Design review of the part shown in the three views and the two pictorial views. Dimensions are in mm from the part's minimum x, y and z. A direction names the side the tool comes from. Round coordinates to 2 decimals unless told otherwise and drop trailing zeros. Loops run counter-clockwise (first coordinate to the right, second up) from the corner with the lowest first, then second, coordinate; pieces in that order, holes last. Notation, with made-up numbers: M 75,-33.75 L 117,-33.75 A6 ccw 117,-24.75 Z; hole C -11,35 d2. An arc over 180 degrees is marked long. Answer in a Markdown table with one row per item. Add a question column.
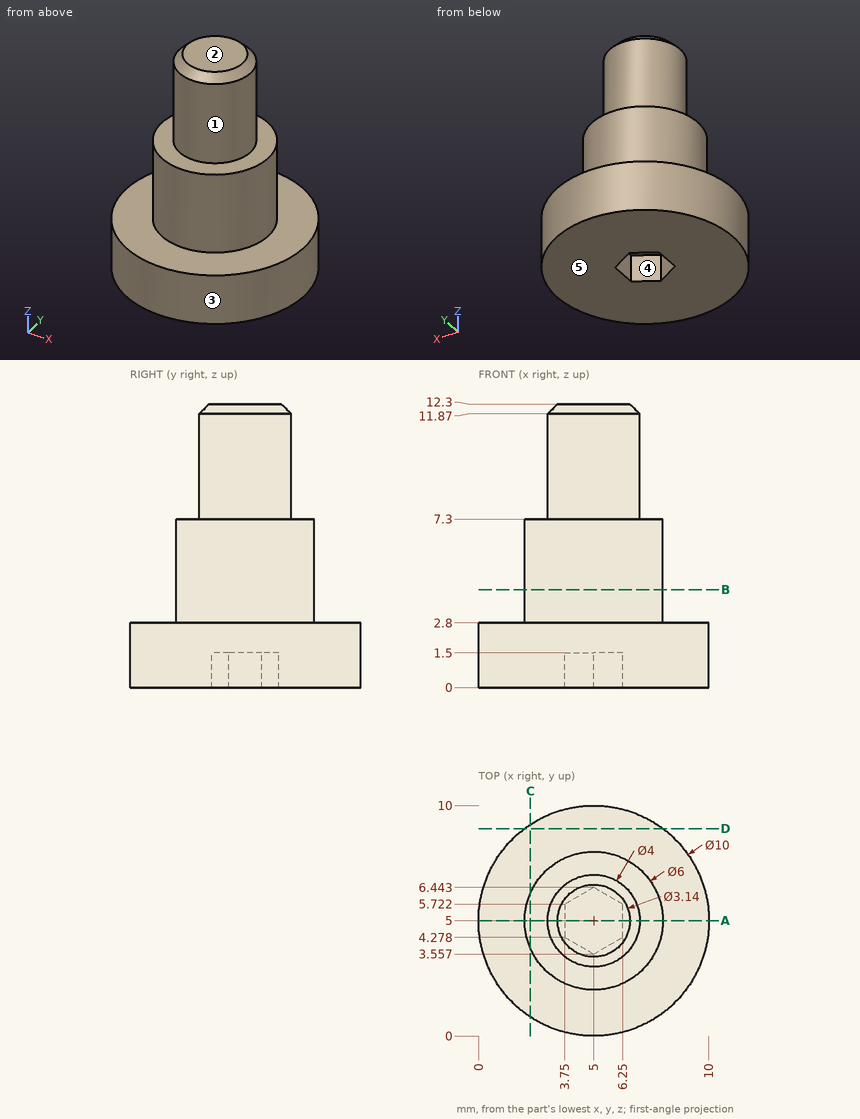
1. To check wall thickness, follow probe 1 along Z at (x, y) = (9.5, 4); probe 2 along Z at (x, y) = (3, 7); probe 3 along X at (y, z) = (5, 6.75). State the ranges of each line that lie inside material, in increasing order.
2. Mouldability with a two-part tool opening along X and no side actions: class the marked faces 3, 4 and 5 as released by +X, released by -X, zero draft, split by the parting line, or undercut.
3. Take a section at B-B, the plane z = 4.25. State the section outline as (x, y) points, and give its area (3 significant figures).
4. Take a section at A-A, the plane y = 5. State the section outline as (x, z) points.
5. For pin 1 Ø2 at (y, z) = (3, 11) entering from +X; pin 2 Ø6 at (x, z) = (8.5, 1.5) entering from -Y (1 decimal); pin 3 Ø5 at (x, z) = (6, 6.5) entering from +Y, all flat-tipped, find the tip position at first contact; note any pin that passes through.
6. Take a section at C-C, the plane x = 2.25. State the section outline as (y, z) points.
7. Machinability: for the marked faces 1 and 2, which of the approach directions +Z, -Z, +X, -X, +Y, -Y give a long, thin tool a straight path to every point of the face, cutting with its end or side? Answer none if there is none.
8. Take a section at D-D, the plane y = 9. State the section outline as (x, z) points.
Check sheet entries:
| question | item | result |
|---|---|---|
| 1 | probe 1 | z = 0 to 2.8 |
| 1 | probe 2 | z = 0 to 7.3 |
| 1 | probe 3 | x = 2 to 8 |
| 2 | face 3 | split by the parting line |
| 2 | face 4 | undercut |
| 2 | face 5 | zero draft |
| 3 | outline | C 5,5 d6 |
| 3 | area | 28.3 mm^2 |
| 4 | outline | M 0,0 L 3.75,0 L 3.75,1.5 L 6.25,1.5 L 6.25,0 L 10,0 L 10,2.8 L 8,2.8 L 8,7.3 L 7,7.3 L 7,11.87 L 6.57,12.3 L 3.43,12.3 L 3,11.87 L 3,7.3 L 2,7.3 L 2,2.8 L 0,2.8 Z |
| 5 | pin 1 | stops at x = 6.73 |
| 5 | pin 2 | stops at y = 0 |
| 5 | pin 3 | stops at y = 8 |
| 6 | outline | M 0.82,0 L 9.18,0 L 9.18,2.8 L 6.2,2.8 L 6.2,7.3 L 3.8,7.3 L 3.8,2.8 L 0.82,2.8 Z |
| 7 | face 1 | +Z |
| 7 | face 2 | +Z, +X, -X, +Y, -Y |
| 8 | outline | M 2,0 L 8,0 L 8,2.8 L 2,2.8 Z |
